Read the model definition and answer for the solid it produces. Units are mm, in the model's axes. A direction names the side the tool comes from. Coordinates: 2 decimals unless noted, no trailing zeros. Loops run counter-clockwise (first coordinate to the right, second up) from the corner with the lowest first, then second, coordinate; pieces in that order, holes last. Notation, with made-up numbers: (-34, 76.5) -> (-13, 76.5) arc R24 ccw to (-13, 87.5) -> close; hole circle Ø9 at (-7, 25.5). An arc over 180 degrees is marked (long way). Answer as a JSON object with one key per item and string values. Group by question number.
1) Consider probe 1 along Y at (x, z) = (0, 4.1); probe 2 along Y at (x, z) = (0, 1.05) (3 decimals); probe 3 along Z at (x, y) = (-3.25, -2.5). Determine where each line is inside the solid, lowest interval first. Write a range as [from, to].
2) Flat-ended cylindrical pins translate along their axes: P1, Ø3, axis at x = 1.5, y = -1, coming from the +Z side; P2, Ø3, axis at x = 7, z = 5.5, coming from the +Y side; P3, Ø4, axis at y = 1, z = 6.5, coming from the +X side. Find the tip coordinate at first contact, or state that the pin passes through.
3) Section A-A, the plane x = 0 is taken. Give the vertices of the cut face in (y, z) (3 decimals), plus the area to 3 significant figures.
4) Which of the six approach directions +Z, -Z, +X, -X, +Y, -Y give full straight-line access (tool end or side, diameter ignored) to faces 1 (the face through (-1, -8, 7.112)), 2 (the face through (-3.3, 1.1, 3.81))?
5) Section D-D, the plane z = 5.75 is taken. Give the vertices of the cut face in (x, y), plus the area to 3 significant figures.
6) Section C-C, the plane z = 0.75 is taken. Give the vertices of the cut face in (x, y) (3 decimals).
from build123d import *

# Parameters (mm, degrees)
SKETCH1_R           = 12.7
SKETCH1_R_2         = 3.175
BOSS_EXTRUDE1_DEPTH = 3.81
SKETCH2_R           = 12.7
SKETCH2_R_2         = 5.08
BOSS_EXTRUDE2_DEPTH = 3.302
FILLET2_R           = 2.54


with BuildPart() as part:
    # Sketch1 → Boss-Extrude1 (new body)
    with BuildSketch(Plane(origin=(0, 0, 0), x_dir=(0, 1, 0), z_dir=(0, 0, 1))):
        with Locations(Location((0, 0, 0), (0, 0, 90))):
            Circle(SKETCH1_R)
        with Locations(Location((0, 0, 0), (0, 0, 90))):
            Circle(SKETCH1_R_2, mode=Mode.SUBTRACT)
    extrude(amount=BOSS_EXTRUDE1_DEPTH)

    # Sketch2 → Boss-Extrude2 (add)
    with BuildSketch(Plane.XY.offset(3.81)):
        with Locations(Location((0, 0, 0), (0, 0, 180))):
            Circle(SKETCH2_R)
        with Locations(Location((0, 0, 0), (0, 0, 180))):
            Circle(SKETCH2_R_2, mode=Mode.SUBTRACT)
    extrude(amount=BOSS_EXTRUDE2_DEPTH)

    # Fillet2
    fillet2_edges = [part.edges().sort_by_distance(p)[0] for p in [
        (12.7, 0, 7.112),
        (5.08, 0, 7.112),
    ]]
    fillet(fillet2_edges, radius=FILLET2_R)


solid = part.part
Determined:
{
 "1": {"probe 1": "[-12.7, -5.08], [5.08, 12.7]", "probe 2": "[-12.7, -3.175], [3.175, 12.7]", "probe 3": "[0, 3.81]"},
 "2": {"P1": "z = 3.81", "P2": "y = 11.37", "P3": "x = 12.7"},
 "3": {"outline": "(-12.7, 0) -> (-3.175, 0) -> (-3.175, 3.81) -> (-5.08, 3.81) -> (-5.08, 4.572) arc R2.54 ccw to (-7.62, 7.112) -> (-10.16, 7.112) arc R2.54 ccw to (-12.7, 4.572) -> close; (3.175, 0) -> (12.7, 0) -> (12.7, 4.572) arc R2.54 ccw to (10.16, 7.112) -> (7.62, 7.112) arc R2.54 ccw to (5.08, 4.572) -> (5.08, 3.81) -> (3.175, 3.81) -> close", "area": "117 mm²"},
 "4": {"face 1": "+Z, +X, -X, +Y, -Y", "face 2": "+Z"},
 "5": {"outline": "circle Ø24.82 at (0, 0); hole circle Ø10.74 at (0, 0)", "area": "393 mm²"},
 "6": {"outline": "circle Ø25.4 at (0, 0); hole circle Ø6.35 at (0, 0)"}
}
